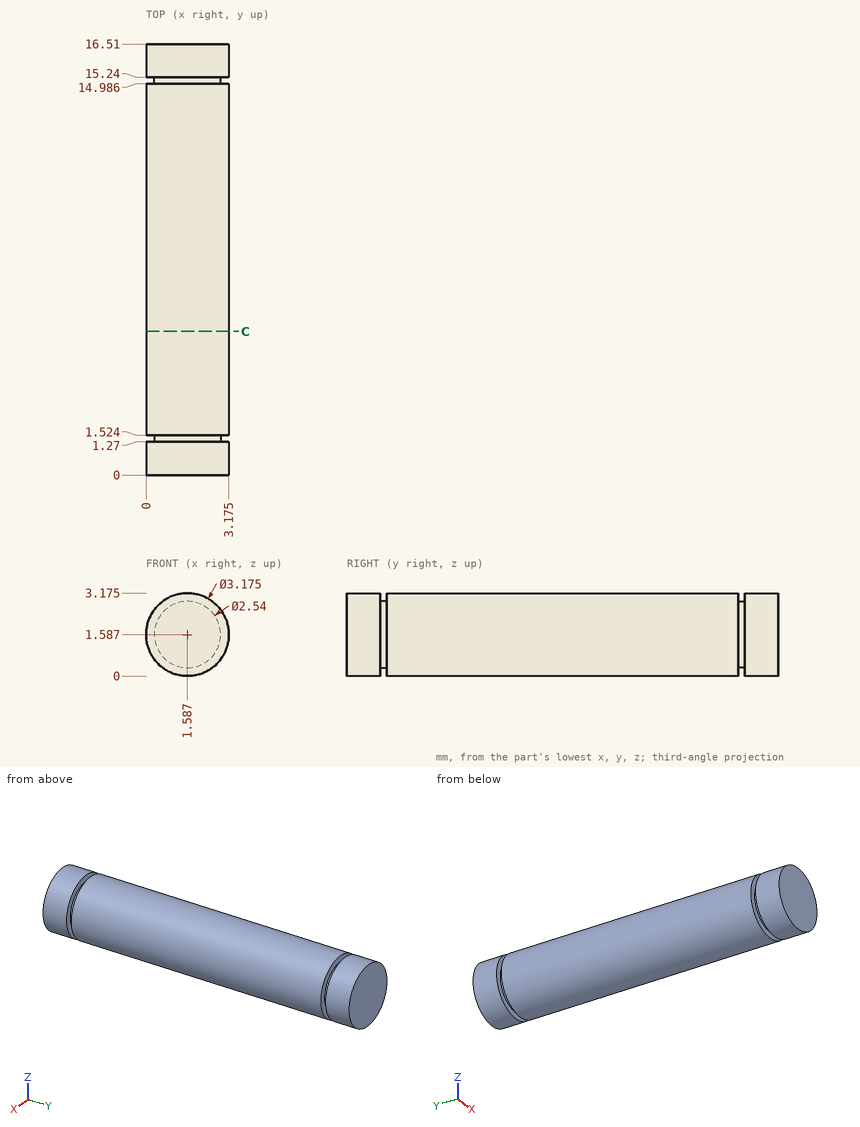
Job drawing, mm, ordinate dimensions from the low corner. One solid piece. Round coordinates to 2 decimals unless told otherwise and drop trailing zeros. Loops run counter-clockwise (first coordinate to the right, second up) from the corner with the lowest first, then second, coordinate; pieces in that order, holes last.
Item 1: Drop a flat-ended pin along its axis: P1, Ø1, axis at y = 11, z = 0.5, coming from the +X side. Give the stop position or say it passes through.
Item 2: Cut at C-C, the plane y = 5.5. Give the cut face in (x, z) (1 decimal).
Item 3: Drill centre lines: line 1 (Y direction, x = 3.05, z = 1.75) (1 decimal); line 2 (Z direction, x = 1.7, y = 14.25) (1 decimal). Where is each one in solid material? Low to high.
A:
1. P1: stops at x = 3.06
2. outline: circle Ø3.2 at (1.6, 1.6)
3. line 1: y = 0 to 1.3, 1.5 to 15, 15.2 to 16.5
3. line 2: z = 0 to 3.2
